Autodesk Inventor part; units mm, degrees
ref_plane "YZ Plane" through (0, 0, 0) normal (1, 0, 0) x (0, 1, 0)
ref_plane "XZ Plane" through (0, 0, 0) normal (0, 1, 0) x (-1, 0, 0)
ref_plane "XY Plane" through (0, 0, 0) normal (0, 0, 1) x (1, 0, 0)
sketch "Sketch1" plane through (0, 0, 0) normal (0, 0, 1) x (1, 0, 0)
  line L0 (0, 0) -> (12, 0)
  line L1 (12, 0) -> (12, 8)
  line L2 (12, 8) -> (0, 8)
  line L3 (0, 8) -> (0, 0)
  line L4 (12, 8) -> (12, 4.75)
  line L5 (12, 4.75) -> (11, 4.75)
  line L6 (11, 4.75) -> (11, 5.75)
  line L7 (11, 5.75) -> (12, 5.75)
  line L8 (0, 5.75) -> (1, 5.75)
  line L9 (1, 5.75) -> (1, 4.75)
  line L10 (1, 4.75) -> (0, 4.75)
  dimension "d0" = 8
  dimension "d1" = 12
  dimension "d2" = 3.25
  dimension "d3" = 2.25
  dimension "d4" = 1
  dimension "d5" = 1
extrude "Extrusion1" add sketch "Sketch1" against normal blind 196.85 contours L3 L10 L9 L8 L2 L1 L7 L6 L5 L0
chamfer "Chamfer1" distance 0.5 angle 45 4 edges at (12, 5.75, -98.425) (12, 4.75, -98.425) (0, 5.75, -98.425) (0, 4.75, -98.425)
chamfer "Chamfer2" distance 0.375 angle 45 2 edges at (12, 8, -98.425) (0, 8, -98.425)
equation "\"d4\" = d5"
properties part number "MGN12"
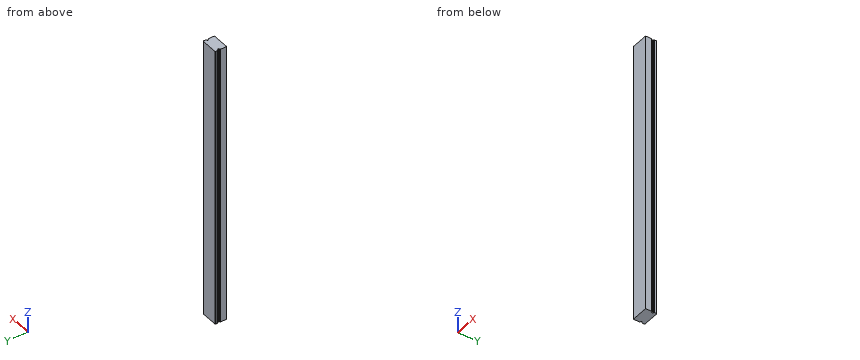
Work out the finished part from the listing and answer in its coordinate system (mm). Round coordinates to 2 decimals unless told otherwise and drop trailing zeros. Write each loop counter-clockwise with the first axis right and the second up, starting at its lowest first coordinate (ties: lowest second). Pieces come first, ordered by that corner, then holes. Notation, with made-up numbers: (8, 78.5) -> (23, 78.5) arc R23 cw to (23, 115.5) -> close; hole circle Ø7 at (28, 44). An arc over 180 degrees is marked (long way). Answer as CSV lines item,"result". Start each with the question number.
(1) Find the intervals of material crossed by probe 1 along Y at (x, z) = (11.25, -181.5); probe 2 along X at (y, z) = (5.5, -169.5), in increasing order.
(2) This flat-tipped pin is pushed along its axis until it touches: pin 1 (1.1 mm diameter, centred on y = 5.5, z = -81, fed in from -X). Where does it stop, or does it pass through?
(3) The part is cut by section A-A, the plane z = -97. Give the vertices of the cut face in (x, y) (3 decimals), then the cut area to 3 significant figures.
Output values:
1,probe 1,"y = 0 to 4.75, 5.75 to 8"
1,probe 2,"x = 1 to 11"
2,pin 1,"stops at x = 0.2"
3,outline,"(0, 0) -> (12, 0) -> (12, 4.25) -> (11.5, 4.75) -> (11, 4.75) -> (11, 5.75) -> (11.5, 5.75) -> (12, 6.25) -> (12, 7.625) -> (11.625, 8) -> (0.375, 8) -> (0, 7.625) -> (0, 6.25) -> (0.5, 5.75) -> (1, 5.75) -> (1, 4.75) -> (0.5, 4.75) -> (0, 4.25) -> close"
3,area,"93.4 mm²"
